from build123d import *

# Parameters (mm, degrees)
F1_DEPTH = 12.7
F3_DEPTH = 50.8
F7_D     = 12.7


with BuildPart() as f1:
    # F0 (on Front) → F1 (new body)
    with BuildSketch(Plane.XZ):
        with BuildLine():
            ThreePointArc((18.115472, 39.387427), (0, 57.502899), (-18.115472, 39.387427))
            Line((-18.115472, 39.387427), (-18.115472, -39.387427))
            ThreePointArc((-18.115472, -39.387427), (0, -21.271955), (18.115472, -39.387427))
            Line((18.115472, -39.387427), (18.115472, 39.387427))
        make_face()
    extrude(amount=-F1_DEPTH)

    # F2 (on face) → F3 (join)
    with BuildSketch(Plane.XZ):
        with BuildLine():
            ThreePointArc((-18.115472, -39.387427), (0, -57.502899), (18.115472, -39.387427))
            ThreePointArc((18.115472, -39.387427), (0, -21.271955), (-18.115472, -39.387427))
        make_face()
    extrude(amount=-F3_DEPTH)

    # F5: F1 across plane


with BuildPart() as f1_1:
    add(f1.part)
    add(f1.part.mirror(Plane.XZ.offset(-50.8)))

    # F7 (through all)
    with Locations(Plane.XZ):
        with Locations((0, -39.387427), (0, 39.387427)):
            Hole(F7_D / 2)


solid = f1_1.part
Source: CAD feature listing. Evaluate the final solid. Frame: model axes, mm. Give positions to 0.01 mm unless a question says otherwise; leave off trailing zeros. Write each loop counter-clockwise with the first axis right and the second up, starting at its lowest first coordinate (ties: lowest second). Pieces come first, ordered by that corner, then holes. Notation, with made-up numbers: (0, -11) -> (46, -11) arc R25 ccw to (46, 20) -> close; hole circle Ø9 at (24.5, 32). An arc over 180 degrees is marked (long way). Return JSON: item names as keys, results as strings. Group by question number.
1. Section D-D, the plane z = -31. Output: boundary loops of the cut face in (x, y).
2. Section C-C, the plane x = 10. Output: boundary loops of the cut face in (y, z).
3. Material intervals for line 1 (Z direction, x = 0, y = 96); line 2 (Y direction, x = -16, z = -18); line 3 (Z direction, x = 0, y = 53), sorted ascending. Write a range as from..to.
4. Mould query, pull axis Z, two halves, no side actions, for faces 1 (the face through (0, 12.7, 10)), 2 (the face through (1.38, 95.34, 33.19)), 3 (the face through (0.4, 6.3, 57.5)). Classes: +Z half, -Z half, draft (parallel to the pull), parting line (faces both ways), or undercut.
5. Pin query (flat end, axial travel): pin 1 Ø10 at (x, y) = (7, 10.5) entering from -Z; pin 2 Ø8 at (y, z) = (18, 43) entering from +X; pin 3 Ø6 at (x, y) = (10.5, 44.5) entering from -Z; pin 4 Ø5 at (x, y) = (-7, 38.5) entering from -Z. Return the tip coordinate at first contact, or that it passes through.
6. Section A-A, the plane x = 0. Output: boundary loops of the cut face in (y, z).
7. Section B-B, the plane y = 46. Output: boundary loops of the cut face in (x, z).
Determined:
{
 "1": {"outline": "(-18.12, 0) -> (18.12, 0) -> (18.12, 12.7) -> (16.06, 12.7) -> (16.06, 88.9) -> (18.12, 88.9) -> (18.12, 101.6) -> (-18.12, 101.6) -> (-18.12, 88.9) -> (-16.06, 88.9) -> (-16.06, 12.7) -> (-18.12, 12.7) -> close"},
 "2": {"outline": "(0, -54.49) -> (101.6, -54.49) -> (101.6, 54.49) -> (88.9, 54.49) -> (88.9, -24.28) -> (12.7, -24.28) -> (12.7, 54.49) -> (0, 54.49) -> close"},
 "3": {"line 1": "z = -57.5..-45.74, -33.04..33.04, 45.74..57.5", "line 2": "y = 0..12.7, 88.9..101.6", "line 3": "z = -57.5..-45.74, -33.04..-21.27"},
 "4": {"face 1": "draft", "face 2": "undercut", "face 3": "+Z half"},
 "5": {"pin 1": "stops at z = -57.39", "pin 2": "passes through", "pin 3": "stops at z = -55.88", "pin 4": "stops at z = -56.94"},
 "6": {"outline": "(0, -57.5) -> (101.6, -57.5) -> (101.6, -45.74) -> (0, -45.74) -> close; (0, -33.04) -> (101.6, -33.04) -> (101.6, 33.04) -> (88.9, 33.04) -> (88.9, -21.27) -> (12.7, -21.27) -> (12.7, 33.04) -> (0, 33.04) -> close; (0, 45.74) -> (12.7, 45.74) -> (12.7, 57.5) -> (0, 57.5) -> close; (88.9, 45.74) -> (101.6, 45.74) -> (101.6, 57.5) -> (88.9, 57.5) -> close"},
 "7": {"outline": "circle Ø36.23 at (0, -39.39); hole circle Ø12.7 at (0, -39.39)"}
}
